CAD build for the part. Positions are in the model's coordinates, mm. Face numbers are marked on the shaded views. A direction names the side the tool comes from. Give positions to 0.01 mm unless a question says otherwise; leave off trailing zeros. Loops run counter-clockwise (first coordinate to the right, second up) from the corner with the lowest first, then second, coordinate; pieces in that order, holes last. Notation, with made-up numbers: (86.25, 84.5) -> (90.25, 84.5) arc R20 cw to (90.25, 111.5) -> close; hole circle Ø1 at (83, 88). An arc over 180 degrees is marked (long way). Use one line per item in the form item = value.
```python
from build123d import *

# Parameters (mm, degrees)
SKETCH013_R     = 2.1
PAD003_DEPTH    = 22
POCKET005_START = -3.1
POCKET005_DEPTH = 15.8
SKETCH017_R     = 1.7
HOLE003_DEPTH   = 25
POCKET007_START = -10
POCKET007_DEPTH = 8
FILLET026_R     = 2
FILLET027_R     = 2
FILLET028_R     = 2
POCKET026_DEPTH = 10
CHAMFER013_SIZE = 1


with BuildPart() as part:
    # Sketch013 → Pad003 (new body)
    with BuildSketch(Plane.XZ):
        with BuildLine():
            Line((14.55, 4.5), (14.55, 26))
            Line((14.55, 26), (23.05, 26))
            Line((23.05, 26), (23.05, -17.2))
            Line((23.05, -18.9604076401), (23.05, -17.2))
            Line((23.05, -18.9604076401), (21.80520382, -20.20520382))
            ThreePointArc((14.55, -17.2), (17.1735954124, -21.1264880132), (21.80520382, -20.20520382))
            Line((14.55, -17.2), (14.55, -6.2))
            Line((10.4965363624, -3.9236141499), (14.55, -6.2))
            ThreePointArc((12.7, 4.5), (8.3464805229, 1.1388011954), (10.4965363624, -3.9236141499))
            Line((14.55, 4.5), (12.7, 4.5))
        make_face()
        with Locations((12.7, 0)):
            Circle(SKETCH013_R, mode=Mode.SUBTRACT)
    extrude(amount=-PAD003_DEPTH)

    # Sketch015 (on Face11 of Pad003) → Pocket005 (cut)
    with BuildSketch(Plane(origin=(0, 22, 0), x_dir=(1, 0, 0), z_dir=(0, 1, 0)).offset(POCKET005_START)):
        with BuildLine():
            ThreePointArc((18.9449979984, 5), (4.7, 0), (18.9449979984, -5))
            Line((18.9449979984, -5), (23.05, -5))
            Line((23.05, 5), (23.05, -5))
            Line((18.9449979984, 5), (23.05, 5))
        make_face()
    extrude(amount=-POCKET005_DEPTH, mode=Mode.SUBTRACT)

    # Sketch017 → Hole003 (cut)
    with BuildSketch(Plane.XZ):
        with Locations((18.8, -17.2)):
            Circle(SKETCH017_R)
    extrude(amount=-HOLE003_DEPTH, mode=Mode.SUBTRACT)

    # Sketch018 (on Face2 of Hole003) → Pocket007 (cut)
    with BuildSketch(Plane.XZ.offset(POCKET007_START)):
        Polygon((19.05, 26), (14.55, 10.5), (14.55, 26), align=None)
    extrude(amount=-POCKET007_DEPTH, mode=Mode.SUBTRACT)

    # Fillet026
    fillet026_edges = [part.edges().sort_by_distance(p)[0] for p in [
        (14.55, 5, 26),
        (14.55, 20, 26),
    ]]
    fillet(fillet026_edges, radius=FILLET026_R)

    # Fillet027
    fillet027_edges = [part.edges().sort_by_distance(p)[0] for p in [
        (14.55, 11, -7.783155),
        (14.55, 11, 7.783155),
        (18.944998, 11, -5),
        (18.944998, 11, 5),
    ]]
    fillet(fillet027_edges, radius=FILLET027_R)

    # Fillet028
    fillet028_edges = [part.edges().sort_by_distance(p)[0] for p in [
        (14.55, 20.45, -6.2),
        (14.55, 1.55, -6.2),
        (14.55, 1.55, 4.5),
        (14.55, 20.45, 4.5),
    ]]
    fillet(fillet028_edges, radius=FILLET028_R)

    # Sketch051 (on Face22 of Fillet028) → Pocket026 (cut)
    with BuildSketch(Plane(origin=(23.05, 0, 0), x_dir=(0, 0, 1), z_dir=(1, 0, 0))):
        with BuildLine():
            ThreePointArc((22, -3.3), (20.3, -5), (22, -6.7))
            Line((22, -6.7), (26, -6.7))
            Line((26, -3.3), (26, -6.7))
            Line((22, -3.3), (26, -3.3))
        make_face()
    extrude(amount=-POCKET026_DEPTH, mode=Mode.SUBTRACT)

    # Chamfer013
    chamfer013_edges = [part.edges().sort_by_distance(p)[0] for p in [
        (23.05, 1.65, 26),
        (23.05, 14.35, 26),
    ]]
    chamfer(chamfer013_edges, length=CHAMFER013_SIZE)


solid = part.part
```
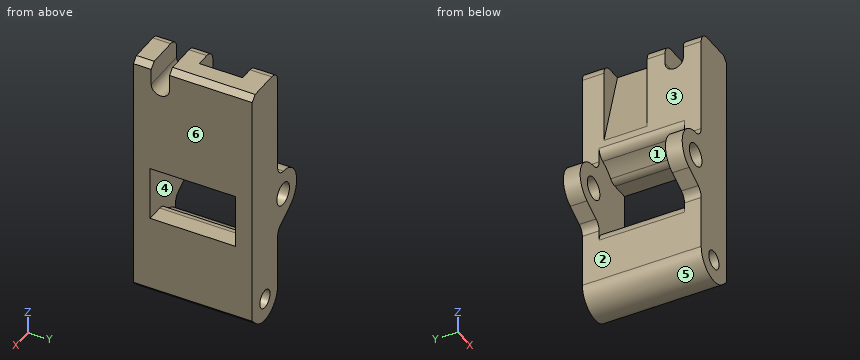
1. Cut at A-A, the plane y = 17.5. Write the cut outline in (x, z).
Result sheet:
outline = (14.55, -17.2) arc R4.25 ccw to (21.81, -20.21) -> (23.05, -18.96) -> (23.05, -5) -> (19.84, -5) arc R2 ccw to (18.41, -5.6) arc R8 cw to (15.78, -7.38) arc R2 ccw to (14.55, -9.23) -> close; (14.55, 9.23) arc R2 ccw to (15.78, 7.38) arc R8 cw to (18.41, 5.6) arc R2 ccw to (19.84, 5) -> (23.05, 5) -> (23.05, 25) -> (22.05, 26) -> (19.05, 26) -> (14.55, 10.5) -> close; hole circle Ø3.4 at (18.8, -17.2)
2. Drill centre lines: line 1 (Y direction, x = 16.75, z = 20.5); line 2 (Z direction, x = 20.75, y = 11.5); line 3 (Z direction, x = 19.75, y = 8.75). Where is each one in solid material? Low to high.
Result sheet:
line_1 = 0 to 4.2, 5.8 to 10, 18 to 22
line_2 = -20.98 to -5, 5 to 26
line_3 = -21.34 to -18.61, -15.79 to -5, 5 to 26
3. Cut at C-C, the plane z = 0. Write the cut outline in (x, y).
Result sheet:
outline = (8.2, 0) -> (10.6, 0) -> (10.6, 3.1) -> (8.2, 3.1) -> close; (8.2, 18.9) -> (10.6, 18.9) -> (10.6, 22) -> (8.2, 22) -> close; (14.8, 0) -> (23.05, 0) -> (23.05, 3.1) -> (14.8, 3.1) -> close; (14.8, 18.9) -> (23.05, 18.9) -> (23.05, 22) -> (14.8, 22) -> close
4. Cut at B-B, the plane x = 9.5. Write the cut outline in (y, z).
Result sheet:
outline = (0, -3.16) -> (3.1, -3.16) -> (3.1, 3.16) -> (0, 3.16) -> close; (18.9, -3.16) -> (22, -3.16) -> (22, 3.16) -> (18.9, 3.16) -> close
5. Tool access for the marked faces 1, 2 and 3: list every direction of +Z, -Z, +X, -X, +Y, -Y with a clear straight run to the whole face (end or side of a thin tool).
Result sheet:
face_1 = -X
face_2 = -Z, -X, +Y, -Y
face_3 = +Z, -X, +Y, -Y
6. Mould opens along Z. For the marked faces 4, 5 and 6 say: pulls with the +Z half, pulls with the -Z half, needs draft (parallel to the pull), parting line crosses it, or undercut.
Result sheet:
face_4 = undercut
face_5 = pulls with the -Z half
face_6 = needs draft
7. Cut at D-D, the plane z = 21. Write the cut outline in (x, y), then the cut area to 3 significant figures.
Result sheet:
outline = (14.55, 0) -> (23.05, 0) -> (23.05, 3.63) -> (14.55, 3.63) -> close; (14.55, 6.37) -> (23.05, 6.37) -> (23.05, 22) -> (14.55, 22) -> (14.55, 18) -> (17.6, 18) -> (17.6, 10) -> (14.55, 10) -> close
area = 139 mm^2
8. Drop flat-ended pins along their axis: P1, Ø10, axis at y = 7.5, z = 14.5, coming from the -X side; P2, Ø1.5, axis at x = 12.5, y = 16.5, coming from the +Z side; P3, Ø3, axis at x = 19, z = 15, coming from the -Y side; P4, Ø1, axis at x = 21, y = 10, coming from the -Z side. Give the stop position or say it passes through.
Result sheet:
P1 = 14.55
P2 = through
P3 = 0
P4 = -21.1
